```python
from build123d import *

# Parameters (mm, degrees)
SKETCH2_R          = 13.92587971
CUT_EXTRUDE1_DEPTH = 25.217488108


with BuildPart() as part:
    # Sketch1 → Revolve1 (revolve)
    with BuildSketch(Plane(origin=(0, 0, 0), x_dir=(0, 0, -1), z_dir=(1, 0, 0)), mode=Mode.PRIVATE) as revolve1_sk:
        with BuildLine():
            Line((0, 0), (36.094855332, 0))
            Line((36.094855332, 0), (36.094855332, 3.8862))
            Line((36.094855332, 3.8862), (20.029355332, 3.8862))
            Line((20.029355332, 3.8862), (20.029355332, 10.16))
            Line((20.029355332, 10.16), (16.600355332, 10.16))
            Line((16.600355332, 10.16), (16.600355332, 4.445))
            Line((16.600355332, 4.445), (10.758355332, 4.064))
            ThreePointArc((10.758355332, 4.064), (5.106033137, 6.448308954), (0, 3.048))
            Line((0, 3.048), (0, 0))
        make_face()
    revolve(revolve1_sk.sketch.rotate(Axis((0, 0, 0), (0, 0, -1)), 180), axis=Axis((0, 0, 0), (0, 0, -1)))

    # Sketch2 → Cut-Extrude1 (cut, through all)
    with BuildSketch(Plane.XY.offset(-16.600355332)):
        Circle(SKETCH2_R)
        Polygon((-3.666174209, 6.35), (3.666174209, 6.35), (7.332348419, 0), (3.666174209, -6.35), (-3.666174209, -6.35), (-7.332348419, 0), align=None, mode=Mode.SUBTRACT)
    extrude(amount=-CUT_EXTRUDE1_DEPTH, mode=Mode.SUBTRACT)


solid = part.part
```
The model under review builds one solid part; all positions refer to its coordinate system, in mm. A direction names the side the tool comes from. Give positions to 0.01 mm unless a question says otherwise; leave off trailing zeros. Loops run counter-clockwise (first coordinate to the right, second up) from the corner with the lowest first, then second, coordinate; pieces in that order, holes last. Notation, with made-up numbers: (67, 53.25) -> (78, 53.25) arc R16 cw to (78, 63.25) -> close; hole circle Ø3 at (-34.75, 54.5). An arc over 180 degrees is marked (long way). Use CSV: the item, a comma, the result in double quotes.
1. Consider section A-A, the plane x = -5. Write out the cut boundary in (y, z) (3 decimals), then the cut area to 3 significant figures.
Result:
outline,"circle Ø8.234 at (0, -5.715); (-4.04, -20.029) -> (4.04, -20.029) -> (4.04, -16.6) -> (-4.04, -16.6) -> close"
area,"81.0 mm²"
2. Consider section D-D, the plane x = 0. Write out the cut boundary in (y, z) (3 decimals), then the cut area to 3 significant figures.
Result:
outline,"(-6.35, -20.029) -> (-3.886, -20.029) -> (-3.886, -36.095) -> (3.886, -36.095) -> (3.886, -20.029) -> (6.35, -20.029) -> (6.35, -16.6) -> (4.445, -16.6) -> (4.064, -10.758) arc R6.477 ccw to (3.048, 0) -> (-3.048, 0) arc R6.477 ccw to (-4.064, -10.758) -> (-4.445, -16.6) -> (-6.35, -16.6) -> close"
area,"339 mm²"
3. Machinability: for faces 1 (the face through (0, -6.35, -18)), 2 (the face through (-3.585, -2.286, -13.638)), 3 (the face through (-5.525, 3.131, -18.291)), which of the approach directions +Z, -Z, +X, -X, +Y, -Y give a long, thin tool a straight path to every point of the face, cutting with its end or side? Answer none if there is none.
Result:
face 1,"-Z, +X, -X, -Y"
face 2,"none"
face 3,"-Z, -X, +Y"
4. To check wall thickness, follow probe 1 along Z at (x, y) = (5.5, 0.75); probe 2 along Z at (x, y) = (0.75, 5.75); probe 3 along Y at (x, z) = (0.25, -27.5). State the ranges of each line that lie inside material, in increasing order. Write a range as from..to.
Result:
probe 1,"z = -20.03..-16.6, -9.05..-2.38"
probe 2,"z = -20.03..-16.6, -8.6..-2.83"
probe 3,"y = -3.88..3.88"
5. Consider section C-C, the plane z = -18.5. Write out the cut boundary in (x, y).
Result:
outline,"(-7.33, 0) -> (-3.67, -6.35) -> (3.67, -6.35) -> (7.33, 0) -> (3.67, 6.35) -> (-3.67, 6.35) -> close"
6. For P1, Ø1.5, axis at x = -5, z = -16.5, coming from the +Y side; P2, Ø1, axis at x = -3, z = -24.5, coming from the +Y side; P3, Ø1, axis at x = -1.5, z = -17.5, coming from the -Y side, all flat-tipped, find the tip position at first contact; note any pin that passes through.
Result:
P1,"stops at y = 5.33"
P2,"stops at y = 2.98"
P3,"stops at y = -6.35"
7. Consider section B-B, the plane y = -5. Write out the cut boundary in (x, z) (3 decimals), then the cut area to 3 significant figures.
Result:
outline,"(-4.446, -20.029) -> (4.446, -20.029) -> (4.446, -16.6) -> (-4.446, -16.6) -> close; circle Ø8.234 at (0, -5.715)"
area,"83.7 mm²"
